```python
from build123d import *

# Parameters (mm, degrees)
SKETCH1_R           = 20
BOSS_EXTRUDE1_DEPTH = 5
SKETCH2_R           = 5.9
BOSS_EXTRUDE2_DEPTH = 45
SKETCH3_R           = 2
CUT_EXTRUDE1_DEPTH  = 5


with BuildPart() as part:
    # Sketch1 → Boss-Extrude1 (new body)
    with BuildSketch(Plane.XY):
        Circle(SKETCH1_R)
    extrude(amount=BOSS_EXTRUDE1_DEPTH)

    # Sketch2 → Boss-Extrude2 (add)
    with BuildSketch(Plane.XY.offset(5)):
        Circle(SKETCH2_R)
    extrude(amount=BOSS_EXTRUDE2_DEPTH)

    # Sketch3 → Cut-Extrude1 (cut)
    with BuildSketch(Plane.XY.offset(5)):
        with Locations((0, 16)):
            Circle(SKETCH3_R)
        with Locations((13.856406461, 8)):
            Circle(SKETCH3_R)
        with Locations((13.856406461, -8)):
            Circle(SKETCH3_R)
        with Locations((0, -16)):
            Circle(SKETCH3_R)
        with Locations((-13.856406461, -8)):
            Circle(SKETCH3_R)
        with Locations((-13.856406461, 8)):
            Circle(SKETCH3_R)
    extrude(amount=-CUT_EXTRUDE1_DEPTH, mode=Mode.SUBTRACT)


solid = part.part
```
Here's how the part is built. I have some questions about the finished solid (model axes, mm). A direction names the side the tool comes from. Round coordinates to 2 decimals unless told otherwise and drop trailing zeros. Order: outer loops, then holes, each group sorted by start corner. A loop starts at its lowest first (then second) coordinate and runs counter-clockwise, first axis right, second up. Notation, with made-up numbers: M 5,-4.5 L 35,-4.5 A21 ccw 35,22.5 Z; hole C 73,84 d9. An arc over 180 degrees is marked long. Answer in a Markdown table with one row per item.
Item 1: For faces 1 (the face through (-5.894, 0.259, 27.185)), 2 (the face through (0, -14, 3)), which set-ups out of +Z, -Z, +X, -X, +Y, -Y let a thin tool reach every point of the face, with its end or its side?
A:
| item | result |
|---|---|
| face 1 | +Z |
| face 2 | +Z, -Z |
Item 2: Imagine slicing it at C-C, the plane y = 8. Write out the boundary of the cut face in (x, z).
A:
| item | result |
|---|---|
| outline | M -18.33,0 L -15.86,0 L -15.86,5 L -18.33,5 Z; M -11.86,0 L 11.86,0 L 11.86,5 L -11.86,5 Z; M 15.86,0 L 18.33,0 L 18.33,5 L 15.86,5 Z |
Item 3: Imagine slicing it at A-A, the plane x = 0. Write out the boundary of the cut face in (y, z).
A:
| item | result |
|---|---|
| outline | M -20,0 L -18,0 L -18,5 L -20,5 Z; M -14,0 L 14,0 L 14,5 L 5.9,5 L 5.9,50 L -5.9,50 L -5.9,5 L -14,5 Z; M 18,0 L 20,0 L 20,5 L 18,5 Z |
Item 4: I'm going to push flat-ended pins straight in: pin 1 (5 mm diameter, centred on x = 0, y = 16, fed in from +Z); pin 2 (3 mm diameter, centred on x = 13.86, y = 8, fed in from +Z); pin 3 (4 mm diameter, centred on y = 4.5, z = 24, fed in from +X); pin 4 (10 mm diameter, centred on y = 7, z = 33.5, fed in from +X). Where does each tip first touch, or does it pass through?
A:
| item | result |
|---|---|
| pin 1 | stops at z = 5 |
| pin 2 | passes through |
| pin 3 | stops at x = 5.34 |
| pin 4 | stops at x = 5.55 |
Item 5: Thinking about a two-plate mould opening in Y: for faces 3 (the face through (0, 0, 50)), 4 (the face through (-14.117, -6.017, 2.535)), 5 (the face through (-4.336, -19.524, 2.465)), which applies, +Y half, -Y half, draft (parallel to the pull), parting line (faces both ways), or undercut?
A:
| item | result |
|---|---|
| face 3 | draft |
| face 4 | undercut |
| face 5 | parting line |
Item 6: If I drill on L1, parallel to X at y = -7.5, z = 4; L2, parallel to Z at x = 7, y = -10.5; L3, parallel to Y at x = -0.5, z = 7, over which ranges is the centre line in solid material (lowest first)? Write a range as from..to.
A:
| item | result |
|---|---|
| L1 | x = -18.54..-15.79, -11.92..11.92, 15.79..18.54 |
| L2 | z = 0..5 |
| L3 | y = -5.88..5.88 |
Item 7: Imagine slicing it at B-B, the plane y = 16. Write out the boundary of the cut face in (x, z).
A:
| item | result |
|---|---|
| outline | M -12,0 L -2,0 L -2,5 L -12,5 Z; M 2,0 L 12,0 L 12,5 L 2,5 Z |
Item 8: Imagine slicing it at D-D, the plane z = 40. Write out the boundary of the cut face in (x, y).
A:
| item | result |
|---|---|
| outline | C 0,0 d11.8 |
